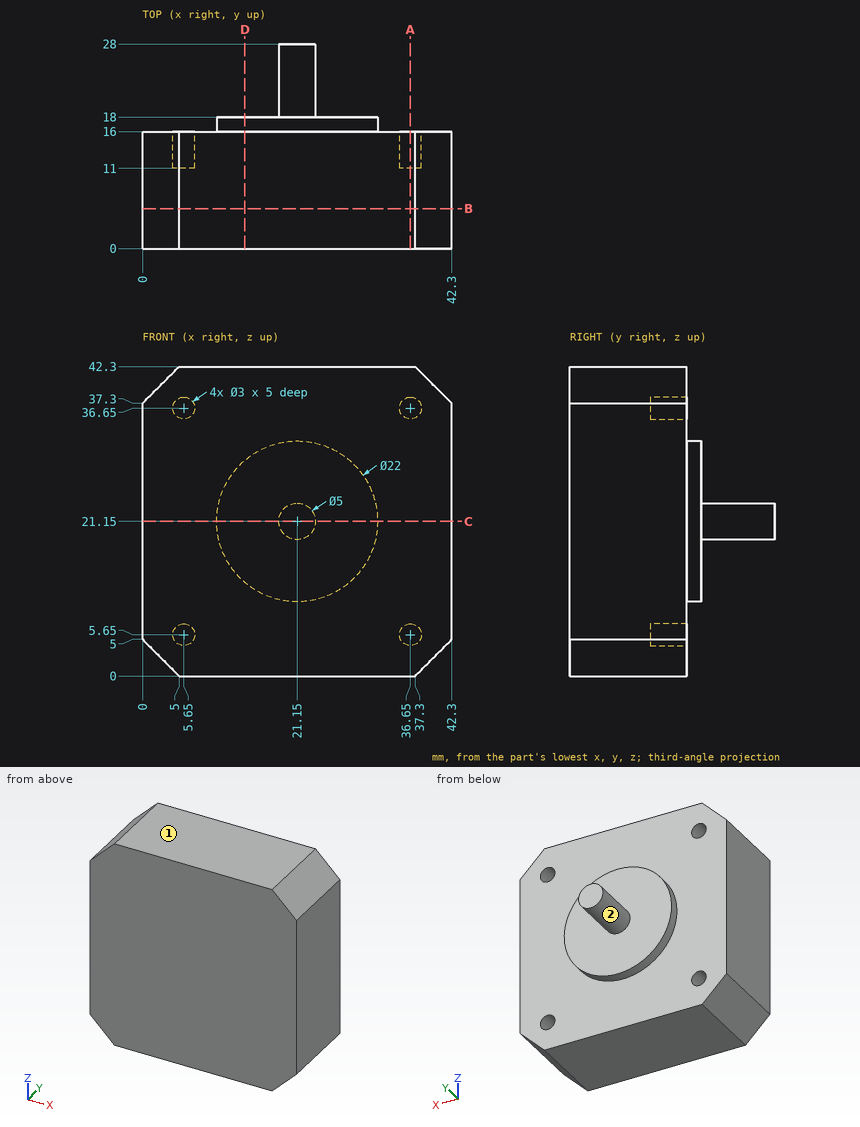
The drawing under review shows one solid part. Ordinate dimensions are in mm from its lowest x, y, z. A direction names the side the tool comes from. Give positions to 0.01 mm unless a question says otherwise; leave off trailing zeros. Order: outer loops, then holes, each group sorted by start corner. A loop starts at its lowest first (then second) coordinate and runs counter-clockwise, first axis right, second up. Notation, with made-up numbers: M 2,83.5 L 48,83.5 A31 cw 48,114.5 Z; hole C 9.5,-1.5 d3. An arc over 180 degrees is marked long. One line per question, with ' | ' between items. Start each with the question number.
Q1. We need section C-C (z = 21.15). Write out the cut boundary in (x, y), plus the area to 3 significant figures.
Q2. Machinability: for the marked faces 1 and 2, which of the approach directions +Z, -Z, +X, -X, +Y, -Y give a long, thin tool a straight path to every point of the face, cutting with its end or side? Answer none if there is none.
Q3. We need section D-D (x = 14). Write out the cut boundary in (y, z), plus the area to 3 significant figures.
Q4. For pin 1 Ø3.5 at (x, z) = (5.65, 36.65) entering from +Y; pin 2 Ø1 at (x, z) = (11.5, 14) entering from -Y; pin 3 Ø2.5 at (x, z) = (36.65, 36.65) entering from +Y; pin 4 Ø6 at (y, z) = (20, 6.5) entering from -X, all flat-tipped, find the tip position at first contact; note any pin that passes through.
Q5. We need section A-A (x = 36.65). Write out the cut boundary in (y, z), plus the area to 3 significant figures.
Q6. We need section B-B (y = 5.5). Write out the cut boundary in (x, z).
Q7. For L1, parallel to X at y = 12, z = 36.65; L2, parallel to Y at x = 20, z = 36; L3, parallel to Y at x = 11, z = 25, list the stretches that pass through material, from the lowest coordinate up. Write a range as [from, to].
Returned:
1) outline: M 0,0 L 42.3,0 L 42.3,16 L 32.15,16 L 32.15,18 L 23.65,18 L 23.65,28 L 18.65,28 L 18.65,18 L 10.15,18 L 10.15,16 L 0,16 Z | area: 771 mm2
2) face 1: +Z, +X, -X, +Y, -Y | face 2: +Y
3) outline: M 0,0 L 16,0 L 16,12.79 L 18,12.79 L 18,29.51 L 16,29.51 L 16,42.3 L 0,42.3 Z | area: 710 mm2
4) pin 1: y = 16 | pin 2: y = 0 | pin 3: y = 11 | pin 4: through
5) outline: M 0,0 L 16,0 L 16,4.15 L 11,4.15 L 11,7.15 L 16,7.15 L 16,35.15 L 11,35.15 L 11,38.15 L 16,38.15 L 16,42.3 L 0,42.3 Z | area: 647 mm2
6) outline: M 0,5 L 5,0 L 37.3,0 L 42.3,5 L 42.3,37.3 L 37.3,42.3 L 5,42.3 L 0,37.3 Z
7) L1: [0, 4.15], [7.15, 35.15], [38.15, 42.3] | L2: [0, 16] | L3: [0, 18]
